Verification items for the finished model (mm, model axes). A direction names the side the tool comes from. Give positions to 0.01 mm unless a question says otherwise; leave off trailing zeros. Write each loop counter-clockwise with the first axis right and the second up, starting at its lowest first coordinate (ties: lowest second). Pieces come first, ordered by that corner, then holes. Notation, with made-up numbers: (47, 4.25) - (75, 4.25) arc R18 ccw to (75, 17.25) - close; hole circle Ø2 at (13, 40). An arc over 180 degrees is marked (long way). Answer as a JSON object with one key per item and string values. Group by question number.
Item 1: Sectioned sample at B-B, the plane x = 7.5. Record the boundary of the cut face in (y, z).
Item 2: Tool access check on faces 4 (the face through (-49.014, -32.419, 23.794)), 5 (the face through (-50, -1, 15)), 6 (the face through (-4, 31, 22)). Record the directions out of +Z, -Z, +X, -X, +Y, -Y that give a thin tool (end or side, any length) a straight path to the whole face; none if there is none.
Item 3: Sectioned sample at D-D, the plane z = 20. Count the separate pieces of the cut face and the enclosed holes in it, and give its area (3 significant figures).
Item 4: Sectioned sample at C-C, the plane z = 26. Record the boundary of the cut face in (x, y).
Item 5: Go/stop test with a flat-tipped pin: pin 1 (14.5 mm diameter, centred on y = -30, z = 20, fed in from -X). Record where the tip stops, or that it passes through.
Item 6: Draft check along Y on faces 1 (the face through (-1, 60, 20)), 2 (the face through (-49.014, -2.419, 23.794)), 3 (the face through (-48.4, 26.9, 40)). Enter one of: +Y half, -Y half, draft (parallel to the pull), parting line (faces both ways), or undercut.
Item 7: Scan lines: line 1 along X through (y, z) = (10, 16); line 2 along Y through (x, z) = (23, 35.5); line 3 along Y through (x, z) = (-18, 16). Record each from-to range of solid material in increasing order. Write a range as [from, to].
Item 8: Sectioned sample at A-A, the plane y = -30. Record the boundary of the cut face in (x, z).
```python
from build123d import *

# Parameters (mm, degrees)
F0_W      = 100
F0_H      = 120
F1_DEPTH  = 40
F2_W      = 96
F2_H      = 116
F3_DEPTH  = 37
F4_R      = 4.5
F5_DEPTH  = 2
F6_W      = 12
F6_H      = 116
F7_DEPTH  = 37
F8_W      = 8
F8_H      = 116
F9_DEPTH  = 37
F10_W     = 12
F10_H     = 10
F11_DEPTH = 37
F12_W     = 42
F12_H     = 53
F13_DEPTH = 37
F14_W     = 42
F14_H     = 51
F15_DEPTH = 37


with BuildPart() as f1:
    # F0 (on Top) → F1 (new body)
    with BuildSketch(Plane.XY):
        Rectangle(F0_W, F0_H)
    extrude(amount=F1_DEPTH)

    # F2 (on face) → F3 (cut)
    with BuildSketch(Plane.XY.offset(40)):
        Rectangle(F2_W, F2_H)
    extrude(amount=-F3_DEPTH, mode=Mode.SUBTRACT)

    # F4 (on face) → F5 (cut)
    with BuildSketch(Plane(origin=(-50, 0, 0), x_dir=(0, -1, 0), z_dir=(-1, 0, 0))):
        with Locations((0, 20)):
            Circle(F4_R)
        with Locations((-30, 20)):
            Circle(F4_R)
        with Locations((30, 20)):
            Circle(F4_R)
    extrude(amount=-F5_DEPTH, mode=Mode.SUBTRACT)

    # F6 (on face) → F7 (join)
    with BuildSketch(Plane.XY.offset(3)):
        Rectangle(F6_W, F6_H)
    extrude(amount=F7_DEPTH)

    # F8 (on face) → F9 (cut)
    with BuildSketch(Plane.XY.offset(40)):
        Rectangle(F8_W, F8_H)
    extrude(amount=-F9_DEPTH, mode=Mode.SUBTRACT)

    # F10 (on face) → F11 (cut)
    with BuildSketch(Plane.XY.offset(40)):
        Rectangle(F10_W, F10_H)
    extrude(amount=-F11_DEPTH, mode=Mode.SUBTRACT)

    # F12 (on face) → F13 (join)
    with BuildSketch(Plane.XY.offset(40)):
        with Locations((27, 31.5)):
            Rectangle(F12_W, F12_H)
    extrude(amount=-F13_DEPTH)

    # F14 (on face) → F15 (cut)
    with BuildSketch(Plane.XY.offset(40)):
        with Locations((27, 32.5)):
            Rectangle(F14_W, F14_H)
    extrude(amount=-F15_DEPTH, mode=Mode.SUBTRACT)


solid = f1.part
```
Geometry check:
{
 "1": {"outline": "(-60, 0) - (60, 0) - (60, 40) - (58, 40) - (58, 3) - (7, 3) - (7, 40) - (5, 40) - (5, 3) - (-58, 3) - (-58, 40) - (-60, 40) - close"},
 "2": {"face 4": "-X", "face 5": "+Z, -Z, -X, +Y, -Y", "face 6": "+Z"},
 "3": {"separate pieces": "3", "enclosed holes": "1", "area": "1,320 mm^2"},
 "4": {"outline": "(-50, -60) - (50, -60) - (50, 60) - (-50, 60) - close; hole (-48, -58) - (-6, -58) - (-6, -5) - (-4, -5) - (-4, -58) - (4, -58) - (4, -5) - (6, -5) - (6, -58) - (48, -58) - (48, 5) - (4, 5) - (4, 58) - (-4, 58) - (-4, 5) - (-6, 5) - (-6, 58) - (-48, 58) - close; hole (6, 7) - (48, 7) - (48, 58) - (6, 58) - close"},
 "5": {"pin 1": "x = -50"},
 "6": {"face 1": "+Y half", "face 2": "undercut", "face 3": "draft"},
 "7": {"line 1": "[-50, -48], [-6, -4], [4, 6], [48, 50]", "line 2": "[-60, -58], [5, 7], [58, 60]", "line 3": "[-60, -58], [58, 60]"},
 "8": {"outline": "(-50, 0) - (50, 0) - (50, 40) - (48, 40) - (48, 3) - (6, 3) - (6, 40) - (4, 40) - (4, 3) - (-4, 3) - (-4, 40) - (-6, 40) - (-6, 3) - (-48, 3) - (-48, 15.5) - (-50, 15.5) - close; (-50, 24.5) - (-48, 24.5) - (-48, 40) - (-50, 40) - close"}
}
